from build123d import *

# Parameters (mm, degrees)
SKETCH_1_W          = 30
SKETCH_1_H          = 40
SKETCH_1_W_2        = 26
SKETCH_1_H_2        = 36
EXTRUDE_1_DEPTH     = 43
SKETCH_2_R          = 2.15
CUT_EXTRUDE_1_DEPTH = 66.946948375
CUT_EXTRUDE_2_REACH = 67.947
SKETCH_3_R          = 17.525
CUT_EXTRUDE_3_REACH = 67.947
SKETCH_4_R          = 10.525
SKETCH_4_R_2        = 2


with BuildPart() as part:
    # 草图1 → 凸台-拉伸1 (new body)
    with BuildSketch(Plane(origin=(0, 0, 0), x_dir=(1, 0, 0), z_dir=(0, 1, 0))):
        with Locations((15, -20)):
            Rectangle(SKETCH_1_W, SKETCH_1_H)
        with Locations((15, -20)):
            Rectangle(SKETCH_1_W_2, SKETCH_1_H_2, mode=Mode.SUBTRACT)
    extrude(amount=EXTRUDE_1_DEPTH)

    # 草图2 → 切除-拉伸1 (cut, through all)
    with BuildSketch(Plane(origin=(0, 0, 0), x_dir=(-1, 0, 0), z_dir=(0, 0, -1))):
        with Locations((-6, 6.5)):
            Circle(SKETCH_2_R)
        with Locations((-24, 6.5)):
            Circle(SKETCH_2_R)
        with Locations((-24, 36.5)):
            Circle(SKETCH_2_R)
        with Locations((-6, 36.5)):
            Circle(SKETCH_2_R)
    extrude(amount=-CUT_EXTRUDE_1_DEPTH, mode=Mode.SUBTRACT)

    # 草图3 → 切除-拉伸2 (cut, up to next)
    with BuildSketch(Plane.ZY, mode=Mode.PRIVATE) as cut_extrude_2_sk1:
        with Locations((20, 21.5)):
            Circle(SKETCH_3_R)
    cut_extrude_2_tool1 = extrude(cut_extrude_2_sk1.sketch, amount=-CUT_EXTRUDE_2_REACH, mode=Mode.PRIVATE) & part.part
    add(cut_extrude_2_tool1.solids().sort_by_distance((0, 21.5, 20))[0], mode=Mode.SUBTRACT)

    # 草图4 → 切除-拉伸3 (cut, up to next)
    with BuildSketch(Plane(origin=(30, 0, 0), x_dir=(0, 0, -1), z_dir=(1, 0, 0)), mode=Mode.PRIVATE) as cut_extrude_3_sk1:
        with Locations((-20, 21.5)):
            Circle(SKETCH_4_R)
    cut_extrude_3_tool1 = extrude(cut_extrude_3_sk1.sketch, amount=-CUT_EXTRUDE_3_REACH, mode=Mode.PRIVATE) & part.part
    # 草图4 → 切除-拉伸3 (cut, up to next)
    with BuildSketch(Plane(origin=(30, 0, 0), x_dir=(0, 0, -1), z_dir=(1, 0, 0)), mode=Mode.PRIVATE) as cut_extrude_3_sk2:
        with Locations((-6, 21.5)):
            Circle(SKETCH_4_R_2)
    cut_extrude_3_tool2 = extrude(cut_extrude_3_sk2.sketch, amount=-CUT_EXTRUDE_3_REACH, mode=Mode.PRIVATE) & part.part
    # 草图4 → 切除-拉伸3 (cut, up to next)
    with BuildSketch(Plane(origin=(30, 0, 0), x_dir=(0, 0, -1), z_dir=(1, 0, 0)), mode=Mode.PRIVATE) as cut_extrude_3_sk3:
        with Locations((-20, 7.5)):
            Circle(SKETCH_4_R_2)
    cut_extrude_3_tool3 = extrude(cut_extrude_3_sk3.sketch, amount=-CUT_EXTRUDE_3_REACH, mode=Mode.PRIVATE) & part.part
    # 草图4 → 切除-拉伸3 (cut, up to next)
    with BuildSketch(Plane(origin=(30, 0, 0), x_dir=(0, 0, -1), z_dir=(1, 0, 0)), mode=Mode.PRIVATE) as cut_extrude_3_sk4:
        with Locations((-34, 21.5)):
            Circle(SKETCH_4_R_2)
    cut_extrude_3_tool4 = extrude(cut_extrude_3_sk4.sketch, amount=-CUT_EXTRUDE_3_REACH, mode=Mode.PRIVATE) & part.part
    # 草图4 → 切除-拉伸3 (cut, up to next)
    with BuildSketch(Plane(origin=(30, 0, 0), x_dir=(0, 0, -1), z_dir=(1, 0, 0)), mode=Mode.PRIVATE) as cut_extrude_3_sk5:
        with Locations((-20, 35.5)):
            Circle(SKETCH_4_R_2)
    cut_extrude_3_tool5 = extrude(cut_extrude_3_sk5.sketch, amount=-CUT_EXTRUDE_3_REACH, mode=Mode.PRIVATE) & part.part
    add(cut_extrude_3_tool1.solids().sort_by_distance((30, 21.5, 20))[0], mode=Mode.SUBTRACT)
    add(cut_extrude_3_tool2.solids().sort_by_distance((30, 21.5, 6))[0], mode=Mode.SUBTRACT)
    add(cut_extrude_3_tool3.solids().sort_by_distance((30, 7.5, 20))[0], mode=Mode.SUBTRACT)
    add(cut_extrude_3_tool4.solids().sort_by_distance((30, 21.5, 34))[0], mode=Mode.SUBTRACT)
    add(cut_extrude_3_tool5.solids().sort_by_distance((30, 35.5, 20))[0], mode=Mode.SUBTRACT)


solid = part.part
The model under review builds one solid part; all positions refer to its coordinate system, in mm. A direction names the side the tool comes from. Round coordinates to 2 decimals unless told otherwise and drop trailing zeros. Loops run counter-clockwise (first coordinate to the right, second up) from the corner with the lowest first, then second, coordinate; pieces in that order, holes last. Notation, with made-up numbers: (-18, -21.75) - (-9, -21.75) arc R17 ccw to (-9, -2.75) - close; hole circle Ø5 at (2, 0). An arc over 180 degrees is marked (long way). Use CSV: the item, a comma, the result in double quotes.
(1) Take a section at A-A, the plane z = 20. Give the boundary of the cut face in (x, y) (3 decimals).
Working result:
outline,"(0, 0) - (2, 0) - (2, 3.975) - (0, 3.975) - close; (0, 39.025) - (2, 39.025) - (2, 43) - (0, 43) - close; (28, 0) - (30, 0) - (30, 5.5) - (28, 5.5) - close; (28, 9.5) - (30, 9.5) - (30, 10.975) - (28, 10.975) - close; (28, 32.025) - (30, 32.025) - (30, 33.5) - (28, 33.5) - close; (28, 37.5) - (30, 37.5) - (30, 43) - (28, 43) - close"
(2) The part is to be moulded in two halves that separate along X. For faces 3 (the flat face through (1.6, 43, 18.4)), 4 (the flat face through (30, 11.6, 15.8)), 5 (the cylindrical face through (24.28, 8.63, 38.99)), say which applies: pulls with the +X half, pulls with the -X half, needs draft (parallel to the pull), parting line crosses it, or undercut.
Working result:
face 3,"needs draft"
face 4,"pulls with the +X half"
face 5,"undercut"
(3) Take a section at D-D, the plane y = 7.5. State how many separate pieces and enclosed holes the cut face has, plus the area to 3 significant figures.
Working result:
separate pieces,"6"
enclosed holes,"0"
area,"183 mm^2"
(4) Take a section at C-C, the plane x = 6. Give the boundary of the cut face in (y, z), plus the area to 3 significant figures.
Working result:
outline,"(0, 0) - (4.35, 0) - (4.35, 2) - (0, 2) - close; (0, 38) - (4.35, 38) - (4.35, 40) - (0, 40) - close; (8.65, 0) - (34.35, 0) - (34.35, 2) - (8.65, 2) - close; (8.65, 38) - (34.35, 38) - (34.35, 40) - (8.65, 40) - close; (38.65, 0) - (43, 0) - (43, 2) - (38.65, 2) - close; (38.65, 38) - (43, 38) - (43, 40) - (38.65, 40) - close"
area,"138 mm^2"
(5) For line 1 (Y direction, x = 28.5, z = 20) (3 decimals); line 2 (Y direction, x = 6, z = 38.65); line 3 (Z direction, x = 4.5, y = 21), list the stretches that pass through material, from the lowest coordinate up.
Working result:
line 1,"y = 0 to 5.5, 9.5 to 10.975, 32.025 to 33.5, 37.5 to 43"
line 2,"y = 0 to 4.35, 8.65 to 34.35, 38.65 to 43"
line 3,"z = 0 to 2, 38 to 40"
(6) Machinability: for faces 1 (the cylindrical face through (29.014, 8.852, 21.474)), 2 (the flat face through (15, 21, 2)), which of the approach directions +Z, -Z, +X, -X, +Y, -Y give a long, thin tool a straight path to every point of the face, cutting with its end or side? Answer none if there is none.
Working result:
face 1,"+X, -X"
face 2,"+Y, -Y"
(7) Clearance check with flat-ended pins moving along their axes: P1, Ø2.5, axis at x = 24, y = 36.5, coming from the +Z side; P2, Ø10, axis at x = 25.5, z = 30, coming from the +Y side; P3, Ø3, axis at y = 19, z = 34, coming from the -X side. State where each tip first meets the part, or that it passes through.
Working result:
P1,"passes through"
P2,"stops at y = 43"
P3,"stops at x = 28"
(8) Take a section at B-B, the plane x = 21.25. Give the boundary of the cut face in (y, z).
Working result:
outline,"(0, 0) - (43, 0) - (43, 2) - (0, 2) - close; (0, 38) - (43, 38) - (43, 40) - (0, 40) - close"
